Design review of the part built by this model. Coordinates are the model's own, in mm. Face numbers are marked on the shaded views. A direction names the side the tool comes from. Coordinates: 2 decimals unless noted, no trailing zeros. Write each loop counter-clockwise with the first axis right and the second up, starting at its lowest first coordinate (ties: lowest second). Pieces come first, ordered by that corner, then holes. Notation, with made-up numbers: (-19.75, 22) - (23.25, 22) arc R13 ccw to (23.25, 47) - close; hole circle Ø11 at (2, -29). An arc over 180 degrees is marked (long way). Answer as CSV lines item,"result". Start each with the question number.
Q1. Machinability: for the marked faces 1 and 2, which of the approach directions +Z, -Z, +X, -X, +Y, -Y give a long, thin tool a straight path to every point of the face, cutting with its end or side? Answer none if there is none.
Q2. We need section D-D (y = 0). Write out the cut boundary in (x, z) (3 decimals), plus the area to 3 significant figures.
Q3. Clearance check with flat-ended pins moving along their axes: pin 1 (1.8 mm diameter, centred on y = -26.1, z = 1.59, fed in from +X); pin 2 (2.5 mm diameter, centred on x = -6, y = 0, fed in from +Z). State where each tip first meets the part, or that it passes through.
Q4. For line 1 along Y through (x, z) = (6, 1.95); line 2 along X through (y, z) = (-13, 2.35); line 3 along Y through (x, z) = (4.25, 1.45), list the stretches that pass through material, from the lowest coordinate up. Write a range as [from, to].
Q5. We need section C-C (x = 6). Write out the cut boundary in (y, z) (3 decimals), plus the area to 3 significant figures.
Q6. We need section B-B (y = -21.9). Write out the cut boundary in (x, z) (1 decimal).
Q7. We need section A-A (z = 1.4). Write out the cut boundary in (x, y).
from build123d import *

# Parameters (mm, degrees)
BOSS_EXTRUDE1_DEPTH         = 3.175
M2_5_CLEARANCE_HOLE1_D      = 2.7
CHAMFER1_SIZE               = 1
TAP_DRILL_FOR_M2X0_4_TAP1_D = 1.6


with BuildPart() as part:
    # Sketch2 → Boss-Extrude1 (new body)
    with BuildSketch(Plane.XY):
        Polygon((-9.82, -6.25), (10, -6.25), (10, 4), (-14.82, 4), (-14.82, -34), (-9.82, -34), align=None)
    extrude(amount=BOSS_EXTRUDE1_DEPTH)

    # M2.5 Clearance Hole1 (through all)
    with Locations(Plane.XY.offset(3.175)):
        with Locations((-6, 0), (6, 0)):
            Hole(M2_5_CLEARANCE_HOLE1_D / 2)

    # Chamfer1
    chamfer1_edges = [part.edges().sort_by_distance(p)[0] for p in [
        (-9.82, -34, 1.5875),
        (-14.82, 4, 1.5875),
        (10, 4, 1.5875),
        (10, -6.25, 1.5875),
        (-9.82, -6.25, 1.5875),
    ]]
    chamfer(chamfer1_edges, length=CHAMFER1_SIZE)

    # Tap Drill for M2x0.4 Tap1 (through all)
    with Locations(Plane.ZY.offset(14.82)):
        with Locations((1.5875, -21.9), (1.5875, -26.1)):
            Hole(TAP_DRILL_FOR_M2X0_4_TAP1_D / 2)


solid = part.part
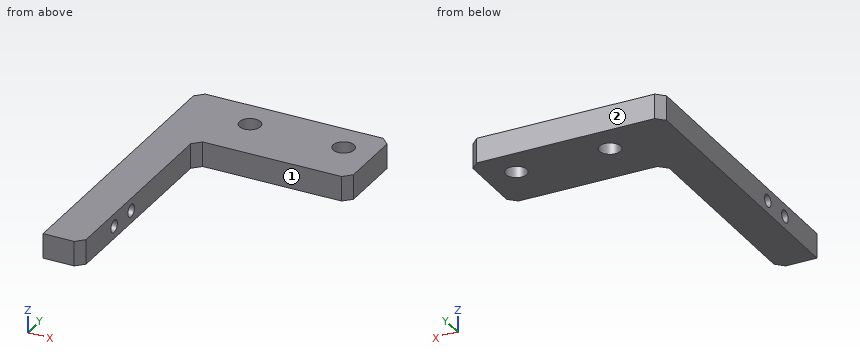
Results list:
1,face 1,"+Z, -Z, +X, -Y"
1,face 2,"+Z, -Z, +X, -X, +Y"
2,outline,"(-14.82, 0) - (-7.35, 0) - (-7.35, 3.175) - (-14.82, 3.175) - close; (-4.65, 0) - (4.65, 0) - (4.65, 3.175) - (-4.65, 3.175) - close; (7.35, 0) - (10, 0) - (10, 3.175) - (7.35, 3.175) - close"
2,area,"61.7 mm2"
3,pin 1,"stops at x = -9.82"
3,pin 2,"passes through"
4,line 1,"y = [-6.25, -1.35], [1.35, 4]"
4,line 2,"x = [-14.82, -9.82]"
4,line 3,"y = [-6.25, 4]"
5,outline,"(-6.25, 0) - (-1.35, 0) - (-1.35, 3.175) - (-6.25, 3.175) - close; (1.35, 0) - (4, 0) - (4, 3.175) - (1.35, 3.175) - close"
5,area,"24.0 mm2"
6,outline,"(-14.8, 0) - (-9.8, 0) - (-9.8, 0.8) - (-14.8, 0.8) - close; (-14.8, 2.4) - (-9.8, 2.4) - (-9.8, 3.2) - (-14.8, 3.2) - close"
7,outline,"(-14.82, -34) - (-10.82, -34) - (-9.82, -33) - (-9.82, -26.88) - (-14.82, -26.88) - close; (-14.82, -25.32) - (-9.82, -25.32) - (-9.82, -22.68) - (-14.82, -22.68) - close; (-14.82, -21.12) - (-9.82, -21.12) - (-9.82, -7.25) - (-8.82, -6.25) - (9, -6.25) - (10, -5.25) - (10, 3) - (9, 4) - (-13.82, 4) - (-14.82, 3) - close; hole circle Ø2.7 at (-6, 0); hole circle Ø2.7 at (6, 0)"
